Autodesk Inventor part; units mm, degrees
ref_plane "YZ Plane" through (0, 0, 0) normal (1, 0, 0) x (0, 1, 0)
ref_plane "XZ Plane" through (0, 0, 0) normal (0, 1, 0) x (-1, 0, 0)
ref_plane "XY Plane" through (0, 0, 0) normal (0, 0, 1) x (1, 0, 0)
sketch "main" plane through (0, 0, 0) normal (0, 0, 1) x (1, 0, 0)
  circle A0 centre (-25.7384, -24.2854) radius 2.1844
  circle A1 centre (-25.7384, 26.5146) radius 2.1844
  circle A2 centre (25.0616, -24.2854) radius 2.1844
  arc A3 (-32.0884, -24.2854) -> (-25.7384, -30.6354) centre (-25.7384, -24.2854) ccw
  arc A4 (25.0616, -30.6354) -> (29.5518, -19.7953) centre (25.0616, -24.2854) ccw
  arc A5 (-21.2482, 31.0047) -> (-32.0884, 26.5146) centre (-25.7384, 26.5146) ccw
  line L0 (-25.7384, -30.6354) -> (25.0616, -30.6354)
  line L1 (-32.0884, -24.2854) -> (-32.0884, 26.5146)
  line L2 (29.5518, -19.7953) -> (-21.2482, 31.0047)
  line L3 (-19.3884, 11.1843) -> (9.7314, -17.9354)
  line L4 (9.7314, -17.9354) -> (-19.3884, -17.9354)
  line L5 (-19.3884, -17.9354) -> (-19.3884, 11.1843)
  circle A6 centre (-25.7384, -11.5854) radius 2.0955
  circle A7 centre (-25.7384, 1.1146) radius 2.0955
  point P0 (-9.8909, -6.4767)
  point P1 (-28.0498, 28.318)
  dimension "d0" = 12.7
  dimension "d1" = 12.7
  dimension "d2" = 12.7
  dimension "d5" = 12.7
  dimension "d6" = 4.191
  dimension "d7" = 4.191
sketch "Sketch1" plane through (0, 0, 0) normal (0, 1, 0) x (-1, 0, 0)
  circle A0 centre (0, 0) radius 2.1844
  circle A1 centre (0, 50.8) radius 2.1844
  circle A2 centre (50.8, 0) radius 2.1844
  arc A3 (-6.35, 0) -> (0, -6.35) centre (0, 0) ccw
  arc A4 (50.8, -6.35) -> (55.2901, 4.4901) centre (50.8, 0) ccw
  arc A5 (4.4901, 55.2901) -> (-6.35, 50.8) centre (0, 50.8) ccw
  line L0 (0, -6.35) -> (50.8, -6.35)
  line L1 (-6.35, 0) -> (-6.35, 50.8)
  line L2 (55.2901, 4.4901) -> (4.4901, 55.2901)
  line L3 (6.35, 35.4697) -> (35.4697, 6.35)
  line L4 (35.4697, 6.35) -> (6.35, 6.35)
  line L5 (6.35, 6.35) -> (6.35, 35.4697)
  circle A6 centre (0, 12.7) radius 2.0955
  circle A7 centre (0, 25.4) radius 2.0955
extrude "Extrusion1" add sketch "Sketch1" along normal blind 1.5875
properties part number "triangle_gusset"
The listing builds one solid part. Answer for the finished solid, in the listing's coordinates (mm). A direction names the side the tool comes from. Round coordinates to 2 decimals unless told otherwise and drop trailing zeros. Loops run counter-clockwise (first coordinate to the right, second up) from the corner with the lowest first, then second, coordinate; pieces in that order, holes last.
1) Consider line 1 (Z direction, x = 0, y = 1.05); line 2 (X direction, y = 0.1, z = -2); line 3 (Z direction, x = -29, y = 0.8). Determine where each line is inside the solid, lowest interval first.
Outcome:
line 1: z = -6.35 to -2.18, 2.18 to 10.6, 14.8 to 23.3, 27.5 to 48.62, 52.98 to 57.15
line 2: x = -56.83 to -51.68, -49.92 to -0.88, 0.88 to 6.03
line 3: z = -6.35 to 6.35, 12.82 to 30.78
2) A cutting plane is placed at B-B on z = 29. Determine the outline of the cut face in (x, y).
Outcome:
outline: (-30.78, 0) - (-12.82, 0) - (-12.82, 1.59) - (-30.78, 1.59) - close; (-6.35, 0) - (6.35, 0) - (6.35, 1.59) - (-6.35, 1.59) - close
3) For faces 4 (the face through (-21, 1, 6.35)), 5 (the face through (4.44, 0.78, -4.54)), determine the directions among +Z, -Z, +X, -X, +Y, -Y from which every point of the face is accessible in a straight line to the end or side of a thin tool.
Outcome:
face 4: +Y, -Y
face 5: -Z, +X, +Y, -Y
4) A cutting plane is placed at D-D on z = 12.7. Determine the outline of the cut face in (x, y).
Outcome:
outline: (-47.08, 0) - (-29.12, 0) - (-29.12, 1.59) - (-47.08, 1.59) - close; (-6.35, 0) - (-2.1, 0) - (-2.1, 1.59) - (-6.35, 1.59) - close; (2.1, 0) - (6.35, 0) - (6.35, 1.59) - (2.1, 1.59) - close
5) A cutting plane is placed at A-A on y = 0.35. Determine the outline of the cut face in (x, z), plus the area to 3 significant figures.
Outcome:
outline: (-55.29, 4.49) arc R6.35 ccw to (-50.8, -6.35) - (0, -6.35) arc R6.35 ccw to (6.35, 0) - (6.35, 50.8) arc R6.35 ccw to (-4.49, 55.29) - close; hole circle Ø4.37 at (-50.8, 0); hole (-35.47, 6.35) - (-6.35, 6.35) - (-6.35, 35.47) - close; hole circle Ø4.37 at (0, 0); hole circle Ø4.37 at (0, 50.8); hole circle Ø4.19 at (0, 12.7); hole circle Ø4.19 at (0, 25.4)
area: 2,020 mm2
6) For a pull along X with two mould halves and no side action, classify faces 1 (the face through (2.526, 0.783, 56.626)), 2 (the face through (-6.35, 1, 21)), 3 (the face through (-18, 1.588, 26)) as released by +X, released by -X, zero draft, split by the parting line, or undercut.
Outcome:
face 1: split by the parting line
face 2: undercut
face 3: zero draft
7) A cutting plane is placed at C-C on x = -17. Determine the outline of the cut face in (y, z), plus the area to 3 significant figures.
Outcome:
outline: (0, -6.35) - (1.59, -6.35) - (1.59, 6.35) - (0, 6.35) - close; (0, 24.82) - (1.59, 24.82) - (1.59, 42.78) - (0, 42.78) - close
area: 48.7 mm2
